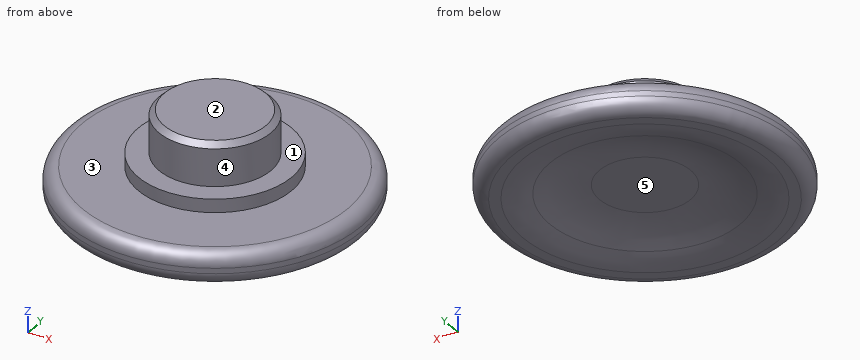
```python
from build123d import *

# Parameters (mm, degrees)
F0_R     = 10.95
F1_DEPTH = 2.4
F2_R     = 4.2
F3_DEPTH = 4.2
F4_R     = 1
F5_R     = 5.75
F5_R_2   = 4.2
F6_DEPTH = 1
F7_R     = 1
F8_R     = 8
F9_DEPTH = 1
F11_SIZE = 0.4
F12_R    = 6


# Not quite as in the source:
# - a fillet or chamfer that OpenCascade refuses, or shapes differently, is made with other operations: its cross-section is extruded or revolved along the edge and cut away or added


with BuildPart() as f1:
    # F0 (on Top) → F1 (new body)
    with BuildSketch(Plane.XY):
        Circle(F0_R)
    extrude(amount=F1_DEPTH)

    # F2 (on face) → F3 (join)
    with BuildSketch(Plane.XY.offset(2.4)):
        Circle(F2_R)
    extrude(amount=F3_DEPTH)

    # F4
    f4_edges = [f1.edges().sort_by_distance(p)[0] for p in [
        (-10.95, 0, 2.4),
    ]]
    fillet(f4_edges, radius=F4_R)

    # F5 (on face) → F6 (join)
    with BuildSketch(Plane.XY.offset(2.4)):
        Circle(F5_R)
        Circle(F5_R_2, mode=Mode.SUBTRACT)
    extrude(amount=F6_DEPTH)

    # F7
    f7_edges = [f1.edges().sort_by_distance(p)[0] for p in [
        (-10.95, 0, 0),
    ]]
    fillet(f7_edges, radius=F7_R)

    # F8 (on face) → F9 (cut)
    with BuildSketch(Plane(origin=(0, 0, 0), x_dir=(1, 0, 0), z_dir=(0, 0, -1))):
        Circle(F8_R)
    extrude(amount=-F9_DEPTH, mode=Mode.SUBTRACT)

    # F10: fillet of radius 11 on 1 edges, made by hand

    # F10_s1 → F10_t2 (revolve)
    with BuildSketch(Plane.XZ):
        with BuildLine():
            ThreePointArc((8, 0), (5.762632185, 0.7470926301), (3.417424305, 1))
            Line((3.417424305, 1), (8, 1))
            Line((8, 1), (8, 0))
        make_face()
    revolve(axis=Axis((0, 0, 1), (0, 0, -1)))

    # F11
    f11_edges = [f1.edges().sort_by_distance(p)[0] for p in [
        (-4.2, 0, 6.6),
    ]]
    chamfer(f11_edges, length=F11_SIZE)

    # F12
    f12_edges = [f1.edges().sort_by_distance(p)[0] for p in [
        (-8, 0, 0),
    ]]
    fillet(f12_edges, radius=F12_R)


solid = f1.part
```
The model under review builds one solid part; all positions refer to its coordinate system, in mm. Face numbers are marked on the shaded views. A direction names the side the tool comes from. Round coordinates to 2 decimals unless told otherwise and drop trailing zeros. Write each loop counter-clockwise with the first axis right and the second up, starting at its lowest first coordinate (ties: lowest second). Pieces come first, ordered by that corner, then holes. Notation, with made-up numbers: (46, -26) - (74, -26) arc R27 cw to (74, 2) - close; hole circle Ø11 at (44, 76.5). An arc over 180 degrees is marked (long way). Answer as CSV lines item,"result". Start each with the question number.
(1) Draft analysis for pull direction X (two halves, no side actions). For the marked faces 3, 4 and 5, state which applies: pulls with the +X half, pulls with the -X half, needs draft (parallel to the pull), parting line crosses it, or undercut.
(2) To check wall thickness, follow line 1 (Z direction, x = -9.25, y = 0.5); line 2 (Z direction, x = 3, y = 0); line 3 (X direction, y = 3.5, z = 6.25). State the ranges of each line that lie inside material, in increasing order.
(3) For pin 1 Ø1 at (y, z) = (-4.5, 2) entering from -X; pin 2 Ø2 at (x, y) = (-5, -2) entering from -Z; pin 3 Ø1.5 at (x, y) = (2.5, 4.5) entering from +Z, all flat-tipped, find the tip position at first contact; note any pin that passes through.
(4) For the marked faces 1 and 2, list the 3-axis set-ups (+Z, -Z, +X, -X, +Y, -Y) from which the entire face can be reached by the end or side of a thin tool; tool diameter is ignored.
(5) We need section A-A on z = 2.75. State the section outline as (x, y) points.
(6) We need section B-B on z = 5.75. State the section outline as (x, y) points, plus the area to 3 significant figures.
Worked answers:
1,face 3,"needs draft"
1,face 4,"parting line crosses it"
1,face 5,"undercut"
2,line 1,"0 to 2.4"
2,line 2,"1 to 6.6"
2,line 3,"-2.23 to 2.23"
3,pin 1,"x = -10.1"
3,pin 2,"z = 0.59"
3,pin 3,"z = 3.4"
4,face 1,"+Z"
4,face 2,"+Z, +X, -X, +Y, -Y"
5,outline,"circle Ø11.5 at (0, 0)"
6,outline,"circle Ø8.4 at (0, 0)"
6,area,"55.4 mm²"
